```python
from build123d import *

# Parameters (mm, degrees)
F1_DEPTH = 24.765
F2_R     = 6.35
F3_R     = 3.175
F4_DEPTH = 127.001
F5_R     = 3.175
F6_DEPTH = 127.001


with BuildPart() as f1:
    # F0 (on Right) → F1 (new body)
    with BuildSketch(Plane.YZ):
        Polygon((4.318, 0), (0, 0), (0, -127), (127, -127), (127, -122.682), (4.318, -122.682), align=None)
    extrude(amount=F1_DEPTH)

    # F2
    f2_edges = [f1.edges().sort_by_distance(p)[0] for p in [
        (12.3825, 4.318, -122.682),
        (12.3825, 0, -127),
    ]]
    fillet(f2_edges, radius=F2_R)

    # F3 (on face) → F4 (cut, through all)
    with BuildSketch(Plane.XZ):
        with Locations((15.113, -104.775)):
            Circle(F3_R)
        with Locations((9.525, -60.325)):
            Circle(F3_R)
        with Locations((15.113, -10.795)):
            Circle(F3_R)
    extrude(amount=-F4_DEPTH, mode=Mode.SUBTRACT)

    # F5 (on face) → F6 (cut, through all)
    with BuildSketch(Plane(origin=(0, 0, -127), x_dir=(1, 0, 0), z_dir=(0, 0, -1))):
        with Locations((9.652, -116.205)):
            Circle(F5_R)
        with Locations((15.24, -66.675)):
            Circle(F5_R)
        with Locations((9.652, -22.225)):
            Circle(F5_R)
    extrude(amount=-F6_DEPTH, mode=Mode.SUBTRACT)


solid = f1.part
```
Geometry check sheet. Reference: the model listing, model coordinates, mm. A direction names the side the tool comes from. Coordinates: 2 decimals unless noted, no trailing zeros. Order: outer loops, then holes, each group sorted by start corner. A loop starts at its lowest first (then second) coordinate and runs counter-clockwise, first axis right, second up. Notation, with made-up numbers: M 74,52 L 81,52 A8 cw 81,67 Z; hole C -20.75,1 d6. An arc over 180 degrees is marked long. One line per question, with ' | ' between items. Start each with the question number.
Item 1: Gauge pin test, flat ends, axial feed: pin 1 (1.5 mm diameter, centred on x = 21.5, y = 25.5, fed in from +Z); pin 2 (1.5 mm diameter, centred on x = 3.5, z = -36, fed in from +Y). Record the tip position at first contact, or that the pin passes through.
Item 2: Cross-section at A-A on x = 10. Enter the section's corners in (y, z).
Item 3: Set-up check for faces 1 (the cylindrical face through (8.964, 119.304, -124.871)), 2 (the flat face through (12, 70, -122.682)): record each of +Z, -Z, +X, -X, +Y, -Y from which the full face is reachable in a straight line by a thin tool's end or side.
Item 4: Cross-section at C-C on y = 45.5. Enter the section's corners in (x, z) (3 decimals), then the cut area to 3 significant figures.
Item 5: Draft check along X on faces 3 (the flat face through (9, 66, -127)), 4 (the cylindrical face through (18.046, 2.129, -12.011)), 5 (the flat face through (24.765, 35, -124)), 6 (the flat face through (0, 35, -124)). Enter one of: pulls with the +X half, pulls with the -X half, needs draft (parallel to the pull), parting line crosses it, or undercut.
Item 6: Cross-section at B-B on z = -29. Enter the section's corners in (x, y) (3 decimals), then the cut area to 3 significant figures.
Item 7: Material ranges on L1, parallel to Y at x = 14.5, z = -65; L2, parallel to Z at x = 22.75, y = 44; L3, parallel to Z at x = 12.75, y = 10, recorded low to high. Write a range as [from, to].
Findings:
1) pin 1: stops at z = -122.68 | pin 2: stops at y = 4.32
2) outline: M 0,-120.65 A6.35 ccw 6.35,-127 L 19.07,-127 L 19.07,-122.68 L 10.67,-122.68 A6.35 cw 4.32,-116.33 L 4.32,-63.46 L 0,-63.46 Z; M 0,-57.19 L 4.32,-57.19 L 4.32,0 L 0,0 Z; M 25.38,-127 L 113.05,-127 L 113.05,-122.68 L 25.38,-122.68 Z; M 119.36,-127 L 127,-127 L 127,-122.68 L 119.36,-122.68 Z
3) face 1: +Z, -Z | face 2: +Z, +X, -X, +Y
4) outline: M 0,-127 L 24.765,-127 L 24.765,-122.682 L 0,-122.682 Z | area: 107 mm²
5) face 3: needs draft | face 4: undercut | face 5: pulls with the +X half | face 6: pulls with the -X half
6) outline: M 0,0 L 24.765,0 L 24.765,4.318 L 0,4.318 Z | area: 107 mm²
7) L1: y = [0, 4.32] | L2: z = [-127, -122.68] | L3: z = [-127, -122.65]
